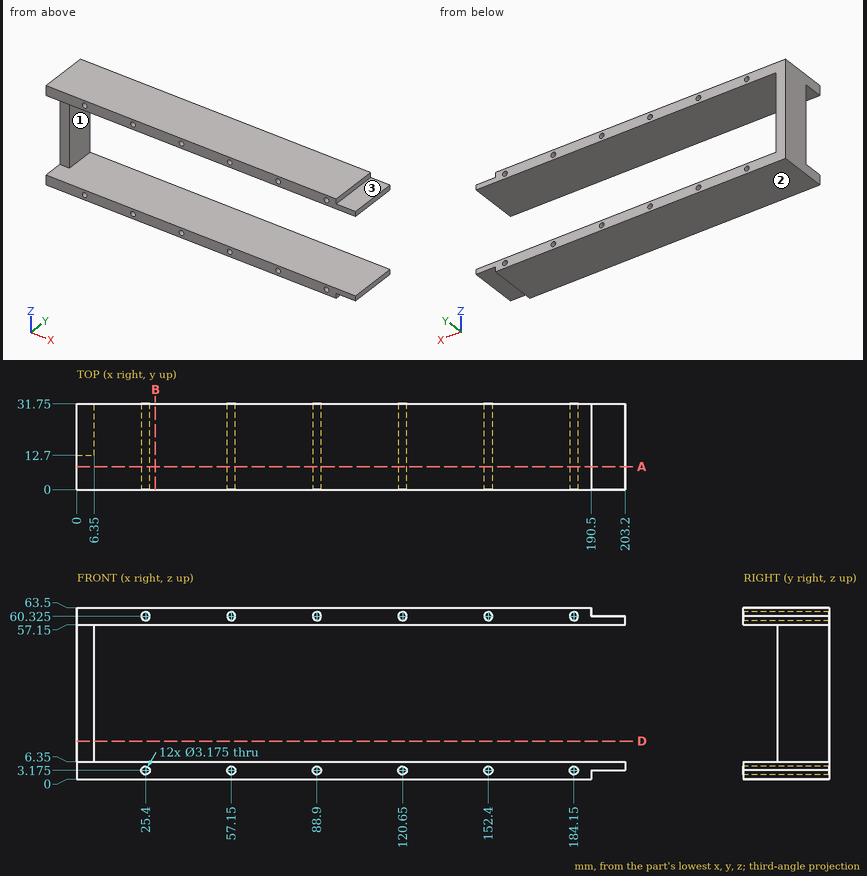
The figure shows three views and two pictorial views of one solid part (mm, origin at its lowest corner). Answer the questions. Coordinates: 2 decimals unless noted, no trailing zeros. Loops run counter-clockwise (first coordinate to the right, second up) from the corner with the lowest first, then second, coordinate; pieces in that order, holes last. Notation, with made-up numbers: (38.25, -30) -> (64.25, -30) arc R17 ccw to (64.25, -16) -> close; hole circle Ø11 at (19, 4). An arc over 180 degrees is marked (long way). Use one line per item in the form item = value. Start each with the question number.
Item 1: The part is cut by section B-B on x = 29. Determine the outline of the cut face in (y, z), then the cut area to 3 significant figures.
Item 2: Flat-ended cylindrical pins translate along their axes: pin 1 Ø6 at (y, z) = (9, 31) entering from +X; pin 2 Ø12 at (y, z) = (15.5, 13) entering from +X; pin 3 Ø3.5 at (y, z) = (21.5, 62.5) entering from +X; pin 4 Ø5 at (x, z) = (4.5, 33) entering from -Y. Find the tip coordinate at first contact, or state that the pin passes through.
Item 3: The mould has two halves that part along Z. Classify the marked faces 1, 2 and 3: released by +Z, released by -Z, zero draft, split by the parting line, or undercut.
Item 4: The part is cut by section A-A on y = 8.5. Count the separate pieces of the cut face and the enclosed holes in it, then the cut area to 3 significant figures.
Item 5: Consider L1, parallel to Z at x = 152.4, y = 14; L2, parallel to Z at x = 47, y = 29. Determine where each line is inside the solid, lowest interval first. Write a range as [from, to].
Item 6: The part is cut by section D-D on z = 14. Determine the outline of the cut face in (x, y), then the cut area to 3 significant figures.
Answer key:
q1.outline = (0, 0) -> (31.75, 0) -> (31.75, 6.35) -> (0, 6.35) -> close; (0, 57.15) -> (31.75, 57.15) -> (31.75, 63.5) -> (0, 63.5) -> close
q1.area = 403 mm2
q2.pin_1 = through
q2.pin_2 = 6.35
q2.pin_3 = 190.5
q2.pin_4 = 12.7
q3.face_1 = undercut
q3.face_2 = released by -Z
q3.face_3 = released by +Z
q4.separate_pieces = 2
q4.enclosed_holes = 12
q4.area = 2,400 mm2
q5.L1 = [0, 1.59], [4.76, 6.35], [57.15, 58.74], [61.91, 63.5]
q5.L2 = [0, 6.35], [57.15, 63.5]
q6.outline = (0, 12.7) -> (6.35, 12.7) -> (6.35, 31.75) -> (0, 31.75) -> close
q6.area = 121 mm2
